from build123d import *

# Parameters (mm, degrees)
SKETCH1_R                  = 1.905
BASE_FLANGE1_DEPTH         = 1.6
SKETCHED_START             = -76.2
SKETCHED_BEND1_OUTLINE_W   = 76.2
SKETCHED_BEND1_OUTLINE_H   = 1.6
SKETCHED_BEND1_DEPTH       = 36.5
SKETCHED_START_2           = 39.7
SKETCHED_BEND1_2_OUTLINE_W = 76.2
SKETCHED_BEND1_2_OUTLINE_H = 1.6
SKETCHED_BEND1_2_DEPTH     = 36.5
SKETCHED_START_3           = -39.7
SKETCHED_BEND1_3_OUTLINE_R = 1.905
SKETCHED_BEND1_3_DEPTH     = 2.3366
SKETCHED_START_4           = 37.3634
SKETCHED_BEND1_4_OUTLINE_R = 1.905
SKETCHED_BEND1_4_DEPTH     = 2.3366
SKETCHED_START_5           = -38.441087378
SKETCHED_BEND1_5_OUTLINE_W = 76.2
SKETCHED_BEND1_5_OUTLINE_H = 1.6
SKETCHED_BEND1_5_DEPTH     = 0.341087378
SKETCHED_START_6           = 38.1
SKETCHED_BEND1_6_OUTLINE_W = 76.2
SKETCHED_BEND1_6_OUTLINE_H = 1.6
SKETCHED_BEND1_6_DEPTH     = 0.341087378
SKETCHED_START_7           = -77
SKETCHED_BEND1_7_DEPTH     = 154
SKETCHED_BEND1_8_DEPTH     = 77
SKETCHED_BEND1_9_DEPTH     = 76.2


with BuildPart() as part:
    # Base-Flange1: sheet metal written as solids
    # Sketch1 → Base-Flange1 (new body)
    with BuildSketch(Plane.XY):
        Polygon((-76.2, 59.69), (-50.8, 59.69), (-50.8, 16.51), (-76.2, 16.51), (-76.2, 0), (-38.1, 0), (-38.1, -76.2), (38.1, -76.2), (38.1, 0), (76.2, 0), (76.2, 16.51), (50.8, 16.51), (50.8, 59.69), (76.2, 59.69), (76.2, 76.2), (-76.2, 76.2), align=None)
        with Locations((-60.96, 63.246)):
            Circle(SKETCH1_R, mode=Mode.SUBTRACT)
        with Locations((-70.866, 63.246)):
            Circle(SKETCH1_R, mode=Mode.SUBTRACT)
        with Locations(Location((-70.866, 12.954, 0), (0, 0, 180))):
            Circle(SKETCH1_R, mode=Mode.SUBTRACT)
        with Locations(Location((-60.96, 12.954, 0), (0, 0, 180))):
            Circle(SKETCH1_R, mode=Mode.SUBTRACT)
        with Locations((60.96, 12.954)):
            Circle(SKETCH1_R, mode=Mode.SUBTRACT)
        with Locations((70.866, 12.954)):
            Circle(SKETCH1_R, mode=Mode.SUBTRACT)
        with Locations(Location((70.866, 63.246, 0), (0, 0, 180))):
            Circle(SKETCH1_R, mode=Mode.SUBTRACT)
        with Locations(Location((60.96, 63.246, 0), (0, 0, 180))):
            Circle(SKETCH1_R, mode=Mode.SUBTRACT)
    extrude(amount=-BASE_FLANGE1_DEPTH)

    # Sketched Bend1: read off the stored shape, not the designer's step
    # Sketched Bend1 outline → Sketched Bend1 (cut)
    with BuildSketch(Plane.YZ.offset(SKETCHED_START)):
        with Locations((38.1, -0.8)):
            Rectangle(SKETCHED_BEND1_OUTLINE_W, SKETCHED_BEND1_OUTLINE_H)
    extrude(amount=SKETCHED_BEND1_DEPTH, mode=Mode.SUBTRACT)

    # Sketched Bend1 2 outline → Sketched Bend1 2 (cut)
    with BuildSketch(Plane.YZ.offset(SKETCHED_START_2)):
        with Locations((38.1, -0.8)):
            Rectangle(SKETCHED_BEND1_2_OUTLINE_W, SKETCHED_BEND1_2_OUTLINE_H)
    extrude(amount=SKETCHED_BEND1_2_DEPTH, mode=Mode.SUBTRACT)

    # Sketched Bend1 3 outline → Sketched Bend1 3 (add)
    with BuildSketch(Plane.YZ.offset(SKETCHED_START_3)):
        Polygon((0, 0), (76.2, 0), (76.2, 37.159514364), (59.69, 37.159514364), (59.69, 11.759514364), (16.51, 11.759514364), (16.51, 37.159514364), (0, 37.159514364), align=None)
        with Locations((12.954, 21.919514364)):
            Circle(SKETCHED_BEND1_3_OUTLINE_R, mode=Mode.SUBTRACT)
        with Locations((63.246, 21.919514364)):
            Circle(SKETCHED_BEND1_3_OUTLINE_R, mode=Mode.SUBTRACT)
        with Locations((12.954, 31.825514364)):
            Circle(SKETCHED_BEND1_3_OUTLINE_R, mode=Mode.SUBTRACT)
        with Locations((63.246, 31.825514364)):
            Circle(SKETCHED_BEND1_3_OUTLINE_R, mode=Mode.SUBTRACT)
    extrude(amount=SKETCHED_BEND1_3_DEPTH)

    # Sketched Bend1 4 outline → Sketched Bend1 4 (add)
    with BuildSketch(Plane.YZ.offset(SKETCHED_START_4)):
        Polygon((0, 0), (76.2, 0), (76.2, 37.159514364), (59.69, 37.159514364), (59.69, 11.759514364), (16.51, 11.759514364), (16.51, 37.159514364), (0, 37.159514364), align=None)
        with Locations((12.954, 21.919514364)):
            Circle(SKETCHED_BEND1_4_OUTLINE_R, mode=Mode.SUBTRACT)
        with Locations((63.246, 21.919514364)):
            Circle(SKETCHED_BEND1_4_OUTLINE_R, mode=Mode.SUBTRACT)
        with Locations((12.954, 31.825514364)):
            Circle(SKETCHED_BEND1_4_OUTLINE_R, mode=Mode.SUBTRACT)
        with Locations((63.246, 31.825514364)):
            Circle(SKETCHED_BEND1_4_OUTLINE_R, mode=Mode.SUBTRACT)
    extrude(amount=SKETCHED_BEND1_4_DEPTH)

    # Sketched Bend1 5 outline → Sketched Bend1 5 (add)
    with BuildSketch(Plane.YZ.offset(SKETCHED_START_5)):
        with Locations((-38.1, -0.8)):
            Rectangle(SKETCHED_BEND1_5_OUTLINE_W, SKETCHED_BEND1_5_OUTLINE_H)
    extrude(amount=SKETCHED_BEND1_5_DEPTH)

    # Sketched Bend1 6 outline → Sketched Bend1 6 (add)
    with BuildSketch(Plane.YZ.offset(SKETCHED_START_6)):
        with Locations((-38.1, -0.8)):
            Rectangle(SKETCHED_BEND1_6_OUTLINE_W, SKETCHED_BEND1_6_OUTLINE_H)
    extrude(amount=SKETCHED_BEND1_6_DEPTH)

    # Sketched Bend1 7 outline → Sketched Bend1 7 (cut)
    with BuildSketch(Plane(origin=(0, 0, 0), x_dir=(1, 0, 0), z_dir=(0, 1, 0)).offset(SKETCHED_START_7)):
        with BuildLine():
            Line((-37.3634, 1.6), (-39.7, 1.6))
            Line((-39.7, 1.6), (-39.7, -0.7366))
            ThreePointArc((-39.7, -0.7366), (-39.015625705, 0.915625705), (-37.3634, 1.6))
        make_face()
        with BuildLine():
            ThreePointArc((-37.3634, 0), (-37.884254855, -0.215745145), (-38.1, -0.7366))
            Line((-38.1, -0.7366), (-38.1, -37.159514364))
            Line((-38.1, -37.159514364), (-37.3634, -37.159514364))
            Line((-37.3634, -37.159514364), (-37.3634, 0))
        make_face()
        with BuildLine():
            ThreePointArc((37.3634, 1.6), (39.015625705, 0.915625705), (39.7, -0.7366))
            Line((39.7, -0.7366), (39.7, 1.6))
            Line((39.7, 1.6), (37.3634, 1.6))
        make_face()
        with BuildLine():
            Line((37.3634, 0), (37.3634, -37.159514364))
            Line((37.3634, -37.159514364), (38.1, -37.159514364))
            Line((38.1, -37.159514364), (38.1, -0.7366))
            ThreePointArc((38.1, -0.7366), (37.884254855, -0.215745145), (37.3634, 0))
        make_face()
    extrude(amount=SKETCHED_BEND1_7_DEPTH, mode=Mode.SUBTRACT)

    # Sketched Bend1 8 outline → Sketched Bend1 8 (cut)
    with BuildSketch(Plane(origin=(0, 0, 0), x_dir=(1, 0, 0), z_dir=(0, 1, 0)).offset(SKETCHED_START_7)):
        Polygon((-37.746292342, 0), (-38.441087378, 1.33663165), (-38.441087378, 0), align=None)
        Polygon((38.441087378, 0), (38.441087378, 1.33663165), (37.746292342, 0), align=None)
    extrude(amount=SKETCHED_BEND1_8_DEPTH, mode=Mode.SUBTRACT)

    # Sketched Bend1 9 outline → Sketched Bend1 9 (add)
    with BuildSketch(Plane(origin=(0, 0, 0), x_dir=(1, 0, 0), z_dir=(0, 1, 0)).offset(SKETCHED_START)):
        with BuildLine():
            Line((-37.3634, 0), (-37.746292342, 0))
            Line((-37.746292342, 0), (-37.703134881, -0.08302539))
            ThreePointArc((-37.703134881, -0.08302539), (-37.538266381, -0.021057333), (-37.3634, 0))
        make_face()
        with BuildLine():
            Line((37.746292342, 0), (37.3634, 0))
            ThreePointArc((37.3634, 0), (37.538266381, -0.021057333), (37.703134881, -0.08302539))
            Line((37.703134881, -0.08302539), (37.746292342, 0))
        make_face()
    extrude(amount=SKETCHED_BEND1_9_DEPTH)


solid = part.part
The model under review builds one solid part; all positions refer to its coordinate system, in mm. A direction names the side the tool comes from. Round coordinates to 2 decimals unless told otherwise and drop trailing zeros. Write each loop counter-clockwise with the first axis right and the second up, starting at its lowest first coordinate (ties: lowest second). Pieces come first, ordered by that corner, then holes. Notation, with made-up numbers: M 19,55.5 L 36,55.5 A7 ccw 36,66.5 Z; hole C 80.5,68.5 d4. An arc over 180 degrees is marked long. Use a Markdown table: item, result. Add a question column.
Q1. We need section A-A, the plane z = 18.5. State the section outline as (x, y) points.
Q2. To check wall thickness, follow line 1 (Z direction, x = -24, y = 17); line 2 (X direction, y = 67, z = 30). State the ranges of each line that lie inside material, in increasing order.
Q3. Machinability: for faces 1 (the face through (-38.1, 38, 11)), 2 (the face through (18, 76.2, -1)), which of the approach directions +Z, -Z, +X, -X, +Y, -Y give a long, thin tool a straight path to every point of the face, cutting with its end or side? Answer none if there is none.
Q4. We need section C-C, the plane y = 29. State the section outline as (x, z) points, plus the area to 3 significant figures.
Q5. The part is to be moulded in two halves that separate along Z. For faces 3 (the face through (38.889, 12.541, 29.966)), 4 (the face through (-38.911, 65.006, 21.19)), 5 (the face through (-1, -1, -1.6)), 6 (the face through (38.1, 38, 11)), say which applies: pulls with the +Z half, pulls with the -Z half, needs draft (parallel to the pull), parting line crosses it, or undercut.
Q6. We need section B-B, the plane z = 4.5. State the section outline as (x, y) points.
Q7. We need section D-D, the plane x = -24.5. State the section outline as (y, z) points.
Q8. Insertion check: pin 1 (1.8 mm diameter, centred on x = 38.5, y = 45.5, fed in from +Z); pin 2 (22.5 mm diameter, centred on x = 3, y = 26.5, fed in from +Z); pin 3 (0.5 mm diameter, centred on x = 39, z = 22, fed in from -Y). Each pin has a flat end and moves straight along its axis. Give the tip position at first contact, or say it passes through.
Findings below:
| question | item | result |
|---|---|---|
| 1 | outline | M -39.7,0 L -38.1,0 L -38.1,16.51 L -39.7,16.51 Z; M -39.7,59.69 L -38.1,59.69 L -38.1,76.2 L -39.7,76.2 Z; M 38.1,0 L 39.7,0 L 39.7,16.51 L 38.1,16.51 Z; M 38.1,59.69 L 39.7,59.69 L 39.7,76.2 L 38.1,76.2 Z |
| 2 | line 1 | z = -1.6 to 0 |
| 2 | line 2 | x = -39.7 to -38.1, 38.1 to 39.7 |
| 3 | face 1 | +Z, +Y, -Y |
| 3 | face 2 | +Z, -Z, +X, -X, +Y |
| 4 | outline | M -39.7,0.74 A2.34 ccw -37.36,-1.6 L 37.36,-1.6 A2.34 ccw 39.7,0.74 L 39.7,11.76 L 38.1,11.76 L 38.1,0.74 A0.74 cw 37.36,0 L -37.36,0 A0.74 cw -38.1,0.74 L -38.1,11.76 L -39.7,11.76 Z |
| 4 | area | 163 mm² |
| 5 | face 3 | undercut |
| 5 | face 4 | undercut |
| 5 | face 5 | pulls with the -Z half |
| 5 | face 6 | needs draft |
| 6 | outline | M -39.7,0 L -38.1,0 L -38.1,76.2 L -39.7,76.2 Z; M 38.1,0 L 39.7,0 L 39.7,76.2 L 38.1,76.2 Z |
| 7 | outline | M -76.2,-1.6 L 76.2,-1.6 L 76.2,0 L -76.2,0 Z |
| 8 | pin 1 | stops at z = 11.76 |
| 8 | pin 2 | stops at z = 0 |
| 8 | pin 3 | stops at y = 0 |
